Can you work these out from the model? Positions are in its coordinate system, mm. Give positions to 0.01 mm unless a question says otherwise; leave off trailing zeros. Write each loop counter-clockwise with the first axis right and the second up, starting at its lowest first coordinate (ties: lowest second). Pieces come first, ordered by that corner, then holes. Notation, with made-up numbers: (50, 8.5) -> (104, 8.5) arc R6 cw to (104, 13.5) -> close; hole circle Ø5 at (33.25, -15.5). An arc over 180 degrees is marked (long way). Answer as CSV lines item,"result". Start each with the question number.
1. I'm going to push flat-ended pins straight in: P1, Ø4.5, axis at x = 600, z = 8.5, coming from the -Y side; P2, Ø8, axis at x = 418, y = -14, coming from the -Z side; P3, Ø6, axis at y = -7.5, z = 10.5, coming from the +X side; P4, Ø3, axis at x = 115, y = -11, coming from the +Z side. Where does each tip first touch, or does it pass through?
2. If we section it at A-A on x = 363.5: Write out the boundary of the cut face in (y, z).
3. I need wall thicknesses on line 1 (Z direction, x = 600, y = -0.9); line 2 (Y direction, x = 507, z = 10); line 3 (Z direction, x = 559.5, y = -18). Which ranges of each line are inside material? Lowest first, please. Write a range as [from, to].
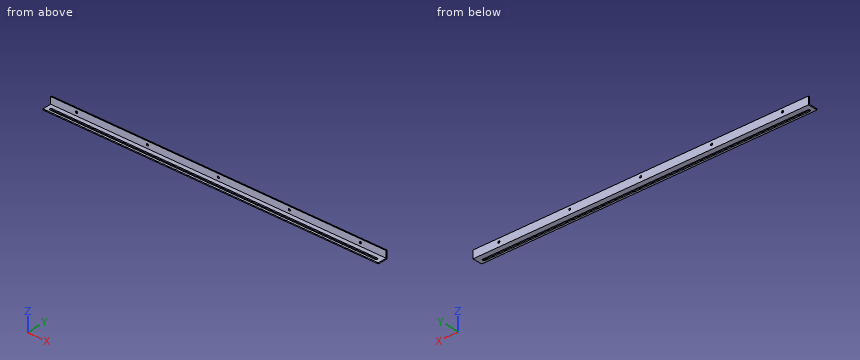
```python
from build123d import *

# Parameters (mm, degrees)
BOSS_EXTRUDE1_DEPTH = 650
CUT_EXTRUDE1_DEPTH  = 2
SKETCH4_R           = 2
CUT_EXTRUDE2_DEPTH  = 2


with BuildPart() as part:
    # Sketch1 → Boss-Extrude1 (new body)
    with BuildSketch(Plane(origin=(0, 0, 0), x_dir=(0, 0, -1), z_dir=(1, 0, 0))):
        Polygon((0, 0), (-15, 0), (-15, -2), (-2, -2), (-2, -19), (0, -19), align=None)
    extrude(amount=BOSS_EXTRUDE1_DEPTH)

    # Sketch3 → Cut-Extrude1 (cut)
    with BuildSketch(Plane(origin=(0, 0, 0), x_dir=(-1, 0, 0), z_dir=(0, 0, -1))):
        with BuildLine():
            Line((-640, -10), (-10, -10))
            ThreePointArc((-10, -10), (-7.5, -12.5), (-10, -15))
            Line((-10, -15), (-640, -15))
            ThreePointArc((-640, -15), (-642.5, -12.5), (-640, -10))
        make_face()
    extrude(amount=-CUT_EXTRUDE1_DEPTH, mode=Mode.SUBTRACT)

    # Sketch4 → Cut-Extrude2 (cut)
    with BuildSketch(Plane.XZ.offset(2)):
        with Locations(Location((325, 8.5, 0), (0, 0, 270))):
            Circle(SKETCH4_R)
        with Locations(Location((187.5, 8.5, 0), (0, 0, 270))):
            Circle(SKETCH4_R)
        with Locations(Location((50, 8.5, 0), (0, 0, 270))):
            Circle(SKETCH4_R)
        with Locations(Location((462.5, 8.5, 0), (0, 0, 270))):
            Circle(SKETCH4_R)
        with Locations(Location((600, 8.5, 0), (0, 0, 270))):
            Circle(SKETCH4_R)
    extrude(amount=-CUT_EXTRUDE2_DEPTH, mode=Mode.SUBTRACT)


solid = part.part
```
Computed values:
1,P1,"stops at y = -2"
1,P2,"stops at z = 0"
1,P3,"passes through"
1,P4,"stops at z = 2"
2,outline,"(-19, 0) -> (-15, 0) -> (-15, 2) -> (-19, 2) -> close; (-10, 0) -> (0, 0) -> (0, 15) -> (-2, 15) -> (-2, 2) -> (-10, 2) -> close"
3,line 1,"z = [0, 6.5], [10.5, 15]"
3,line 2,"y = [-2, 0]"
3,line 3,"z = [0, 2]"
